```python
from build123d import *

# Parameters (mm, degrees)
SKETCH_1_R            = 6.78
EXTRUDE_2_DEPTH       = 11
SKETCH_3_R            = 9
EXTRUDE_355_DEPTH     = 1.5
SKETCH_4_R            = 9
EXTRUDE_447_DEPTH     = 10.5
SKETCH_5_R            = 2.525
CUT_EXTRUDE_536_DEPTH = 24


with BuildPart() as part:
    # 草图1 → 凸台-拉伸2 (new body)
    with BuildSketch(Plane(origin=(0, 0, 0), x_dir=(1, 0, 0), z_dir=(0, 1, 0))):
        Circle(SKETCH_1_R)
    extrude(amount=EXTRUDE_2_DEPTH)

    # 草图3 → Extrude 355 (add)
    with BuildSketch(Plane(origin=(0, 11, 0), x_dir=(1, 0, 0), z_dir=(0, 1, 0))):
        Circle(SKETCH_3_R)
    extrude(amount=EXTRUDE_355_DEPTH)

    # 草图4 → Extrude 447 (add)
    with BuildSketch(Plane.XZ):
        Circle(SKETCH_4_R)
    extrude(amount=EXTRUDE_447_DEPTH)

    # 草图5 → Cut-Extrude 536 (cut, through all)
    with BuildSketch(Plane.XZ.offset(10.5)):
        Circle(SKETCH_5_R)
    extrude(amount=-CUT_EXTRUDE_536_DEPTH, mode=Mode.SUBTRACT)


solid = part.part
```
Can you work these out from the model? Positions are in its coordinate system, mm. A direction names the side the tool comes from. Coordinates: 2 decimals unless noted, no trailing zeros. Loops run counter-clockwise (first coordinate to the right, second up) from the corner with the lowest first, then second, coordinate; pieces in that order, holes last.
Item 1: Suppose I cut it at D-D (x = -5). Please give me the cut outline in (y, z), then the cut area to 3 significant figures.
Answers below:
outline: (-10.5, -7.48) - (0, -7.48) - (0, -4.58) - (11, -4.58) - (11, -7.48) - (12.5, -7.48) - (12.5, 7.48) - (11, 7.48) - (11, 4.58) - (0, 4.58) - (0, 7.48) - (-10.5, 7.48) - close
area: 280 mm2
Item 2: Suppose I cut it at C-C (y = -7.25). Please give me the cut outline in (x, z) (3 decimals), then the cut area to 3 significant figures.
Answers below:
outline: circle Ø18 at (0, 0); hole circle Ø5.05 at (0, 0)
area: 234 mm2
Item 3: Please list where these lines run through material, in increasing order: L1, parallel to Y at x = -7.5, z = 3.75; L2, parallel to Z at x = 0, y = -1 (3 decimals); L3, parallel to Z at x = 0, y = 7.5 (3 decimals).
Answers below:
L1: y = -10.5 to 0, 11 to 12.5
L2: z = -9 to -2.525, 2.525 to 9
L3: z = -6.78 to -2.525, 2.525 to 6.78
Item 4: Suppose I cut it at A-A (x = 0). Please give me the cut outline in (y, z) (3 decimals), then the cut area to 3 significant figures.
Answers below:
outline: (-10.5, -9) - (0, -9) - (0, -6.78) - (11, -6.78) - (11, -9) - (12.5, -9) - (12.5, -2.525) - (-10.5, -2.525) - close; (-10.5, 2.525) - (12.5, 2.525) - (12.5, 9) - (11, 9) - (11, 6.78) - (0, 6.78) - (0, 9) - (-10.5, 9) - close
area: 249 mm2
Item 5: Which directions (+Z, -Z, +X, -X, +Y, -Y) give clear straight access to the entire face, cutting with the end or side of a thin tool? Please do faces 4 (the face through (2, 12.5, 2)), 5 (the face through (-0.883, 5.423, -6.722)).
Answers below:
face 4: +Z, -Z, +X, -X, +Y
face 5: none
Item 6: If we mould it in two halves opening along Y, with no side actions, what happens to faces 1 (the face through (1, 0, 7)), 2 (the face through (2, -10.5, -2)), 3 (the face through (-1.172, -5.176, 8.923))? For each: released by +Y, released by -Y, zero draft, split by the parting line, or undercut.
Answers below:
face 1: undercut
face 2: released by -Y
face 3: zero draft
Item 7: I'm going to push flat-ended pins straight in: pin 1 (1.5 mm diameter, centred on y = 2, z = -4.5, fed in from +X); pin 2 (8 mm diameter, centred on y = -2.5, z = 5, fed in from +X); pin 3 (1 mm diameter, centred on y = 10, z = 3, fed in from -X). Where does each tip first touch, or does it pass through?
Answers below:
pin 1: stops at x = 5.65
pin 2: stops at x = 8.94
pin 3: stops at x = -6.3
Item 8: Suppose I cut it at B-B (z = 0). Please give me the cut outline in (x, y) (3 decimals), then the cut area to 3 significant figures.
Answers below:
outline: (-9, -10.5) - (-2.525, -10.5) - (-2.525, 12.5) - (-9, 12.5) - (-9, 11) - (-6.78, 11) - (-6.78, 0) - (-9, 0) - close; (2.525, -10.5) - (9, -10.5) - (9, 0) - (6.78, 0) - (6.78, 11) - (9, 11) - (9, 12.5) - (2.525, 12.5) - close
area: 249 mm2
